For this review, take the finished solid that the model builds, in its own axes (mm). Face numbers are marked on the shaded views. A direction names the side the tool comes from. Give positions to 0.01 mm unless a question says otherwise; leave off trailing zeros. Order: outer loops, then holes, each group sorted by start corner. A loop starts at its lowest first (then second) coordinate and runs counter-clockwise, first axis right, second up.
from build123d import *

# Parameters (mm, degrees)
SKETCH1_W           = 5.8
SKETCH1_H           = 5.8
BOSS_EXTRUDE1_DEPTH = 7
SKETCH3_W           = 2.9
SKETCH3_H           = 2.9
CUT_EXTRUDE1_DEPTH  = 3.8
SKETCH4_W           = 7
SKETCH4_H           = 7
BOSS_EXTRUDE2_DEPTH = 1.7
CHAMFER1_SIZE       = 1.2


with BuildPart() as part:
    # Sketch1 → Boss-Extrude1 (new body)
    with BuildSketch(Plane(origin=(0, 0, 0), x_dir=(1, 0, 0), z_dir=(0, 1, 0))):
        with Locations((2.9, 2.9)):
            Rectangle(SKETCH1_W, SKETCH1_H)
    extrude(amount=BOSS_EXTRUDE1_DEPTH)

    # Sketch3 → Cut-Extrude1 (cut)
    with BuildSketch(Plane(origin=(0, 7, 0), x_dir=(1, 0, 0), z_dir=(0, 1, 0))):
        with Locations((2.9, 2.9)):
            Rectangle(SKETCH3_W, SKETCH3_H)
    extrude(amount=-CUT_EXTRUDE1_DEPTH, mode=Mode.SUBTRACT)

    # Sketch4 → Boss-Extrude2 (add)
    with BuildSketch(Plane.XZ):
        with Locations((2.9, -2.9)):
            Rectangle(SKETCH4_W, SKETCH4_H)
    extrude(amount=BOSS_EXTRUDE2_DEPTH)

    # Chamfer1
    chamfer1_edges = [part.edges().sort_by_distance(p)[0] for p in [
        (-0.6, -1.7, -2.9),
        (2.9, -1.7, -6.4),
        (6.4, -1.7, -2.9),
        (2.9, -1.7, 0.6),
    ]]
    chamfer(chamfer1_edges, length=CHAMFER1_SIZE)


solid = part.part
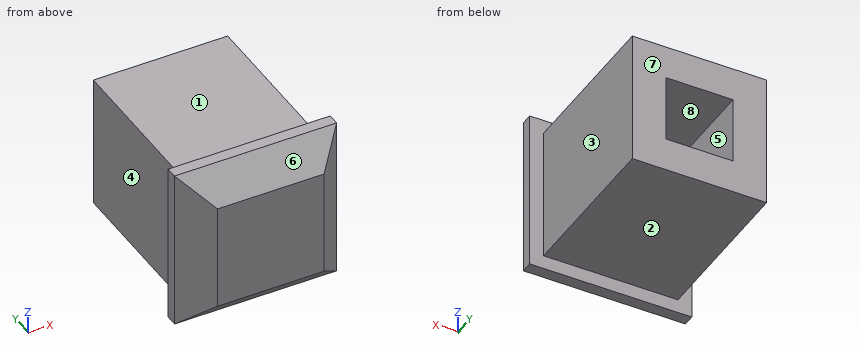
1) Tool access review of the marked faces 1, 2, 3, 4 and 5: name each direction out of +Z, -Z, +X, -X, +Y, -Y from which nothing blocks a thin tool from reaching the whole face with its end or side.
Answer sheet:
face 1: +Z, +X, -X, +Y
face 2: -Z, +X, -X, +Y
face 3: +Z, -Z, +X, +Y
face 4: +Z, -Z, -X, +Y
face 5: +Y
2) We need section B-B on z = -1. Give the boundary of the cut face in (x, y), then the cut area to 3 significant figures.
Answer sheet:
outline: (-0.6, -0.5) - (0.6, -1.7) - (5.2, -1.7) - (6.4, -0.5) - (6.4, 0) - (5.8, 0) - (5.8, 7) - (0, 7) - (0, 0) - (-0.6, 0) - close
area: 51.1 mm2
3) We need section A-A on y = 4.25. Give the boundary of the cut face in (x, z).
Answer sheet:
outline: (0, -5.8) - (5.8, -5.8) - (5.8, 0) - (0, 0) - close; hole (1.45, -4.35) - (4.35, -4.35) - (4.35, -1.45) - (1.45, -1.45) - close
4) We need section C-C on x = 3.5. Give the boundary of the cut face in (y, z).
Answer sheet:
outline: (-1.7, -5.2) - (-0.5, -6.4) - (0, -6.4) - (0, -5.8) - (7, -5.8) - (7, -4.35) - (3.2, -4.35) - (3.2, -1.45) - (7, -1.45) - (7, 0) - (0, 0) - (0, 0.6) - (-0.5, 0.6) - (-1.7, -0.6) - close
5) Draft analysis for pull direction Z (two halves, no side actions). For the marked faces 6, 7 and 8, state which applies: +Z half, -Z half, draft (parallel to the pull), parting line (faces both ways), or undercut.
Answer sheet:
face 6: +Z half
face 7: draft
face 8: undercut
6) Clearance check with flat-ended pins moving along their axes: pin 1 (1.4 mm diameter, centred on x = 3, y = 4, fed in from -Z); pin 2 (0.9 mm diameter, centred on x = 3.5, z = -3, fed in from +Y); pin 3 (1.5 mm diameter, centred on x = 2, y = 5, fed in from +Z); pin 4 (2 mm diameter, centred on x = 4, y = 0.5, fed in from -Z). State where each tip first meets the part, or that it passes through.
Answer sheet:
pin 1: stops at z = -5.8
pin 2: stops at y = 3.2
pin 3: stops at z = 0
pin 4: stops at z = -6.4
7) To check wall thickness, follow line 1 (X direction, y = 4.5, z = -3.5); line 2 (X direction, y = 2, z = -0.5); line 3 (Z direction, x = 1, y = 0.75). State the ranges of each line that lie inside material, in increasing order.
Answer sheet:
line 1: x = 0 to 1.45, 4.35 to 5.8
line 2: x = 0 to 5.8
line 3: z = -5.8 to 0
8) We need section D-D on z = -3.5. Give the boundary of the cut face in (x, y).
Answer sheet:
outline: (-0.6, -0.5) - (0.6, -1.7) - (5.2, -1.7) - (6.4, -0.5) - (6.4, 0) - (5.8, 0) - (5.8, 7) - (4.35, 7) - (4.35, 3.2) - (1.45, 3.2) - (1.45, 7) - (0, 7) - (0, 0) - (-0.6, 0) - close
